Verification items for the finished model (mm, model axes). Coordinates: 2 decimals unless noted, no trailing zeros. Write each loop counter-clockwise with the first axis right and the second up, starting at its lowest first coordinate (ties: lowest second). Pieces come first, ordered by that corner, then holes. Notation, with made-up numbers: (22, 20) -> (58, 20) arc R23 ccw to (58, 39) -> close; hole circle Ø7 at (-28.5, 5). An arc over 180 degrees is marked (long way). Write item = value, one per line. Start each with the question number.
(1) Material ranges on probe 1 along X at (y, z) = (1.75, 167); probe 2 along Z at (x, y) = (1, 2.5); probe 3 along X at (y, z) = (3.25, 189), recorded low to high. Write a range as [from, to].
(2) Section check A-A (x = -13). Record the cut outline in (y, z), plus the area to 3 significant figures.
(3) Gauge pin test, flat ends, axial feed: pin 1 Ø1.8 at (x, y) = (145, 3.5) entering from +Z; pin 2 Ø1.8 at (y, z) = (4.5, 317.5) entering from -X; pin 3 Ø3 at (x, y) = (146.5, 3.5) entering from -Z. Record the tip position at first contact, or that the pin passes through.
(4) Section check C-C (x = -51.5). Record the cut outline in (y, z), plus the area to 3 significant figures.
(5) Section check D-D (y = 5). State how many separate pieces and enclosed holes the cut face has, plus the area to 3 significant figures.
(6) Section check B-B (z = 95). Record the cut outline in (x, y), plus the area to 3 significant figures.
```python
from build123d import *

# Parameters (mm, degrees)
BOSS_EXTRUDE1_DEPTH = 6
SKETCH2_W           = 40
SKETCH2_H           = 40
CUT_EXTRUDE1_DEPTH  = 10
FILLET1_R           = 10
CUT_EXTRUDE4_DEPTH  = 16
FILLET2_R           = 5
FILLET3_R           = 5
CUT_EXTRUDE5_DEPTH  = 16
FILLET4_R           = 5
SKETCH5_W           = 40
SKETCH5_H           = 40
CUT_EXTRUDE6_DEPTH  = 16
FILLET5_R           = 10
SKETCH6_W           = 65
SKETCH6_H           = 30
CUT_EXTRUDE7_DEPTH  = 16
FILLET6_R           = 10


with BuildPart() as part:
    # Sketch1 → Boss-Extrude1 (new body)
    with BuildSketch(Plane(origin=(0, 0, 0), x_dir=(1, 0, 0), z_dir=(0, 1, 0))):
        Polygon((-157.408498061, 145.557138299), (-157.408498061, 72.557138299), (-163.408498061, 72.557138299), (-163.408498061, 32.557138299), (-157.408498061, 32.557138299), (-157.408498061, -115.442861701), (-163.408498061, -115.442861701), (-163.408498061, -155.442861701), (-157.408498061, -155.442861701), (-157.408498061, -228.442861701), (-163.408498061, -228.442861701), (-163.408498061, -268.442861701), (-157.408498061, -268.442861701), (-157.408498061, -341.442861701), (142.591501939, -341.442861701), (142.591501939, -268.442861701), (148.591501939, -268.442861701), (148.591501939, -228.442861701), (142.591501939, -228.442861701), (142.591501939, -155.442861701), (148.591501939, -155.442861701), (148.591501939, -115.442861701), (142.591501939, -115.442861701), (142.591501939, 32.557138299), (148.591501939, 32.557138299), (148.591501939, 72.557138299), (142.591501939, 72.557138299), (142.591501939, 145.557138299), (148.591501939, 145.557138299), (148.591501939, 185.557138299), (142.591501939, 185.557138299), (142.591501939, 258.557138299), (-157.408498061, 258.557138299), (-157.408498061, 185.557138299), (-163.408498061, 185.557138299), (-163.408498061, 145.557138299), align=None)
    extrude(amount=BOSS_EXTRUDE1_DEPTH)

    # Sketch2 → Cut-Extrude1 (cut)
    with BuildSketch(Plane(origin=(0, 6, 0), x_dir=(1, 0, 0), z_dir=(0, 1, 0))):
        with Locations((-97.408498061, -171.800004558)):
            Rectangle(SKETCH2_W, SKETCH2_H)
        with Locations((62.591501939, -171.442861701)):
            Rectangle(SKETCH2_W, SKETCH2_H)
    extrude(amount=-CUT_EXTRUDE1_DEPTH, mode=Mode.SUBTRACT)

    # Fillet1
    fillet1_edges = [part.edges().sort_by_distance(p)[0] for p in [
        (-117.408498061, 3, 191.800004558),
        (-117.408498061, 3, 151.800004558),
        (-77.408498061, 3, 151.800004558),
        (-77.408498061, 3, 191.800004558),
        (42.591501939, 3, 191.442861701),
        (42.591501939, 3, 151.442861701),
        (82.591501939, 3, 151.442861701),
        (82.591501939, 3, 191.442861701),
    ]]
    fillet(fillet1_edges, radius=FILLET1_R)

    # Sketch3 → Cut-Extrude4 (cut)
    with BuildSketch(Plane(origin=(0, 6, 0), x_dir=(1, 0, 0), z_dir=(0, 1, 0))):
        Polygon((-102.408498061, -26.800004558), (-102.408498061, -106.800004558), (-107.408498061, -106.800004558), (-107.408498061, -32.800004558), (-128.408498061, -32.800004558), align=None)
        Polygon((-152.408498061, -106.800004558), (-122.408498061, -106.800004558), (-122.408498061, -46.800004558), (-145.408498061, -46.800004558), (-152.408498061, -26.800004558), align=None)
    extrude(amount=-CUT_EXTRUDE4_DEPTH, mode=Mode.SUBTRACT)

    # Fillet2
    fillet2_edges = [part.edges().sort_by_distance(p)[0] for p in [
        (-107.408498061, 3, 32.800004558),
        (-145.408498061, 3, 46.800004558),
        (-122.408498061, 3, 46.800004558),
    ]]
    fillet(fillet2_edges, radius=FILLET2_R)

    # Fillet3
    fillet3_edges = [part.edges().sort_by_distance(p)[0] for p in [
        (-102.408498061, 3, 106.800004558),
        (-152.408498061, 3, 106.800004558),
        (-122.408498061, 3, 106.800004558),
    ]]
    fillet(fillet3_edges, radius=FILLET3_R - 0.0001)  # a hair under: the kernel refuses the full size

    # Sketch4 → Cut-Extrude5 (cut)
    with BuildSketch(Plane(origin=(0, 6, 0), x_dir=(1, 0, 0), z_dir=(0, 1, 0))):
        Polygon((65.591501939, -41.442861701), (65.591501939, -121.442861701), (95.591501939, -121.442861701), (95.591501939, -61.442861701), (72.591501939, -61.442861701), align=None)
        Polygon((115.591501939, -41.442861701), (89.591501939, -47.442861701), (110.591501939, -47.442861701), (110.591501939, -121.442861701), (115.591501939, -121.442861701), align=None)
    extrude(amount=-CUT_EXTRUDE5_DEPTH, mode=Mode.SUBTRACT)

    # Fillet4
    fillet4_edges = [part.edges().sort_by_distance(p)[0] for p in [
        (115.591501939, 3, 121.442861701),
        (110.591501939, 3, 47.442861701),
        (72.591501939, 3, 61.442861701),
        (95.591501939, 3, 61.442861701),
        (95.591501939, 3, 121.442861701),
        (65.591501939, 3, 121.442861701),
    ]]
    fillet(fillet4_edges, radius=FILLET4_R - 0.0001)  # a hair under: the kernel refuses the full size

    # Sketch5 → Cut-Extrude6 (cut)
    with BuildSketch(Plane(origin=(0, 6, 0), x_dir=(1, 0, 0), z_dir=(0, 1, 0))):
        with Locations((-52.408498061, 88.557138299)):
            Rectangle(SKETCH5_W, SKETCH5_H)
        with Locations((48.591501939, 18.557138299)):
            Rectangle(SKETCH5_W, SKETCH5_H)
    extrude(amount=-CUT_EXTRUDE6_DEPTH, mode=Mode.SUBTRACT)

    # Fillet5
    fillet5_edges = [part.edges().sort_by_distance(p)[0] for p in [
        (-32.408498061, 3, -108.557138299),
        (-32.408498061, 3, -68.557138299),
        (-72.408498061, 3, -68.557138299),
        (-72.408498061, 3, -108.557138299),
        (28.591501939, 3, 1.442861701),
        (28.591501939, 3, -38.557138299),
        (68.591501939, 3, -38.557138299),
        (68.591501939, 3, 1.442861701),
    ]]
    fillet(fillet5_edges, radius=FILLET5_R)

    # Sketch6 → Cut-Extrude7 (cut)
    with BuildSketch(Plane(origin=(0, 6, 0), x_dir=(1, 0, 0), z_dir=(0, 1, 0))):
        with Locations((-7.408498061, 233.557138299)):
            Rectangle(SKETCH6_W, SKETCH6_H)
    extrude(amount=-CUT_EXTRUDE7_DEPTH, mode=Mode.SUBTRACT)

    # Fillet6
    fillet6_edges = [part.edges().sort_by_distance(p)[0] for p in [
        (25.091501939, 3, -248.557138299),
        (25.091501939, 3, -218.557138299),
        (-39.908498061, 3, -218.557138299),
        (-39.908498061, 3, -248.557138299),
    ]]
    fillet(fillet6_edges, radius=FILLET6_R)


solid = part.part
```
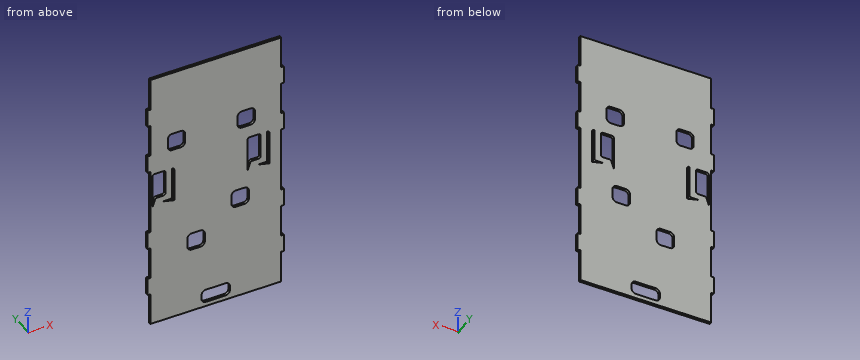
Response:
q1.probe_1 = [-157.41, -117.41], [-77.41, 42.59], [82.59, 142.59]
q1.probe_2 = [-258.56, -248.56], [-218.56, 341.44]
q1.probe_3 = [-157.41, -114.35], [-80.47, 46.04], [79.14, 142.59]
q2.outline = (0, -258.56) -> (6, -258.56) -> (6, -248.56) -> (0, -248.56) -> close; (0, -218.56) -> (6, -218.56) -> (6, 341.44) -> (0, 341.44) -> close
q2.area = 3,420 mm2
q3.pin_1 = 268.44
q3.pin_2 = -157.41
q3.pin_3 = -185.56
q4.outline = (0, -258.56) -> (6, -258.56) -> (6, -108.56) -> (0, -108.56) -> close; (0, -68.56) -> (6, -68.56) -> (6, 341.44) -> (0, 341.44) -> close
q4.area = 3,360 mm2
q5.separate_pieces = 1
q5.enclosed_holes = 9
q5.area = 169,000 mm2
q6.outline = (-157.41, 0) -> (-152.41, 0) -> (-152.41, 6) -> (-157.41, 6) -> close; (-122.41, 0) -> (-107.41, 0) -> (-107.41, 6) -> (-122.41, 6) -> close; (-102.41, 0) -> (65.59, 0) -> (65.59, 6) -> (-102.41, 6) -> close; (95.59, 0) -> (110.59, 0) -> (110.59, 6) -> (95.59, 6) -> close; (115.59, 0) -> (142.59, 0) -> (142.59, 6) -> (115.59, 6) -> close
q6.area = 1,380 mm2
